Read the model definition and answer for the solid it produces. Units are mm, in the model's axes. A direction names the side the tool comes from. Coordinates: 2 decimals unless noted, no trailing zeros. Write each loop counter-clockwise with the first axis right and the second up, starting at its lowest first coordinate (ties: lowest second). Pieces come first, ordered by that corner, then holes.
1) Which of the six approach directions +Z, -Z, +X, -X, +Y, -Y give full straight-line access (tool end or side, diameter ignored) to faces 1 (the face through (0.301, 14.752, 0.285)), 2 (the face through (0.285, 4.248, 0.301)), 3 (the face through (1.875, 3.49, 3.127))?
2) The part is cut by section B-B (y = 9.5). Determine the outline of the cut face in (x, z), then the cut area to 3 significant figures.
3) The part is cut by section D-D (y = 16.25). Determine the outline of the cut face in (x, z), then the cut area to 3 significant figures.
4) The part is cut by section A-A (x = 30). Determine the outline of the cut face in (y, z).
5) The part is cut by section C-C (x = 12). Determine the outline of the cut face in (y, z), then the cut area to 3 significant figures.
6) Each of these flat-tipped pins is pushed along its axis until it touches: pin 1 Ø1.4 at (x, y) = (55, 3.5) entering from +Z; pin 2 Ø1.7 at (x, y) = (25, 14) entering from -Z. Where does it stop, or does it pass through?
7) Find the intervals of material crossed by line 1 (Y direction, x = 56, z = 2.4); line 2 (X direction, y = 13, z = 2.3); line 3 (Y direction, x = 54, z = 4.2), in increasing order.
8) Determine the mould class of faces 4 (the face through (45.875, 8.681, 3.127)), 5 (the face through (60, 9, 3)), 6 (the face through (30.392, 0.285, 0.301)) for opening direction X: +X half, -X half, draft (parallel to the pull), parting line (faces both ways), or undercut.
Autodesk Fusion 360 part; units mm, degrees
sketch "草图1" plane through (0, 0, 0) normal (0, 0, 1) x (1, 0, 0)
  line L0 (0, 0) -> (60, 0)
  line L1 (60, 0) -> (60, 19)
  line L2 (60, 19) -> (0, 19)
  line L3 (0, 19) -> (0, 0)
  line L4 (0, 9.5) -> (60, 9.5) construction
  line L5 (0, 12.44) -> (60, 12.44)
  line L6 (60, 12.44) -> (60, 6.56)
  line L7 (60, 6.56) -> (0, 6.56)
  line L8 (0, 6.56) -> (0, 12.44)
  line L9 (0, 12.44) -> (60, 6.56) construction
  line L10 (60, 12.44) -> (0, 6.56) construction
  point P0 (30, 9.5)
  point P1 (30, 9.5)
  dimension "d1" = 60
  dimension "d2" = 19
  dimension "d3" = 60
  dimension "d4" = 5.88
extrude "拉伸1" add sketch "草图1" along normal blind 5
extrude "拉伸2" add sketch "草图1" against normal blind 1 contours L1 L3 L5 L6 L7 L8
sketch "草图2" plane through (0, 0, 5) normal (0, 0, 1) x (-1, 0, 0)
  line L0 (0, 0) -> (-60, 0)
  line L1 (-60, 0) -> (-60, -19)
  line L2 (-60, -19) -> (0, -19)
  line L3 (0, -19) -> (0, 0)
  point P0 (-30, -9.5)
hole "孔1" at (30, 9.5, 5) direction (0, 0, -1) diameter 3.2 depth 8 tip angle 180 counterbore diameter 6.5 counterbore depth 3.4
sketch "草图4" plane through (0, 0, 5) normal (0, 0, 1) x (-1, 0, 0)
  circle A0 centre (-30, -9.5) radius 3.25
  line L0 (0, 0) -> (-60, 0)
  line L1 (-60, 0) -> (-60, -19)
  line L2 (-60, -19) -> (0, -19)
  line L3 (0, -19) -> (0, 0)
  line L4 (-40.689, -19) -> (-40.689, 3.3911)
  circle A1 centre (-56, -2.6) radius 2.3
  circle A2 centre (-56, -13) radius 2.3
  circle A3 centre (-48, -7.8) radius 2.3
  line L5 (-40.689, 3.3911) -> (-60, 3.3911)
  line L6 (-60, -19) -> (-40.689, -19)
  line L7 (-60, 3.3911) -> (-60, -19)
  line L8 (-19.311, -19) -> (0, -19)
  line L9 (-19.311, 3.3911) -> (-19.311, -19)
  line L10 (0, -19) -> (0, 3.3911)
  line L11 (0, 3.3911) -> (-19.311, 3.3911)
  circle A4 centre (-4, -2.6089) radius 2.3
  circle A5 centre (-12, -7.8089) radius 2.3
  circle A6 centre (-4, -13.0089) radius 2.3
  point P0 (-60, -19)
  point P1 (-60, -19)
  dimension "d14" = 4.6
  dimension "d15" = 4.6
  dimension "d16" = 4.6
  dimension "d17" = 4.6
  dimension "d18" = 4.6
  dimension "d19" = 4.6
extrude "拉伸3" cut sketch "草图4" against normal blind 3.8 contours A1 | A2 | A3 | A4 | A5 | A6
fillet "圆角1" radius 2 4 edges at (60, 0, 2.5) (60, 19, 2.5) (0, 19, 2.5) (0, 0, 2.5)
fillet "圆角2" radius 0.5 4 edges at (60, 9.5, -1) (30, 6.56, -1) (30, 12.44, -1) (0, 9.5, -1)
fillet "圆角3" radius 1 10 edges at (0, 4.28, 0) (0.5858, 0.5858, 0) (30, 0, 0) (59.4142, 0.5858, 0) (60, 4.28, 0) (60, 14.72, 0) (59.4142, 18.4142, 0) (30, 19, 0) (0.5858, 18.4142, 0) (0, 14.72, 0)
Reported:
1. face 1: -Z, -X, +Y
1. face 2: -Z, -X, -Y
1. face 3: +Z
2. outline: (0, -0.5) arc R0.5 ccw to (0.5, -1) - (28.4, -1) - (28.4, 1.6) - (26.75, 1.6) - (26.75, 5) - (13.56, 5) - (13.56, 1.2) - (10.44, 1.2) - (10.44, 5) - (0, 5) - close; (31.6, -1) - (59.5, -1) arc R0.5 ccw to (60, -0.5) - (60, 5) - (49.55, 5) - (49.55, 1.2) - (46.45, 1.2) - (46.45, 5) - (33.25, 5) - (33.25, 1.6) - (31.6, 1.6) - close
2. area: 306 mm2
3. outline: (0, 1) arc R1 ccw to (1, 0) - (59, 0) arc R1 ccw to (60, 1) - (60, 5) - (0, 5) - close
3. area: 300 mm2
4. outline: (0, 1) arc R1 ccw to (1, 0) - (6.56, 0) - (6.56, -0.5) arc R0.5 ccw to (7.06, -1) - (7.9, -1) - (7.9, 1.6) - (6.25, 1.6) - (6.25, 5) - (0, 5) - close; (11.1, -1) - (11.94, -1) arc R0.5 ccw to (12.44, -0.5) - (12.44, 0) - (18, 0) arc R1 ccw to (19, 1) - (19, 5) - (12.75, 5) - (12.75, 1.6) - (11.1, 1.6) - close
5. outline: (0, 1) arc R1 ccw to (1, 0) - (6.56, 0) - (6.56, -0.5) arc R0.5 ccw to (7.06, -1) - (11.94, -1) arc R0.5 ccw to (12.44, -0.5) - (12.44, 0) - (18, 0) arc R1 ccw to (19, 1) - (19, 5) - (10.11, 5) - (10.11, 1.2) - (5.51, 1.2) - (5.51, 5) - (0, 5) - close
5. area: 82.9 mm2
6. pin 1: stops at z = 1.2
6. pin 2: stops at z = 0
7. line 1: y = 0 to 0.3, 4.9 to 10.7, 15.3 to 19
7. line 2: x = 0 to 1.7, 6.3 to 53.7, 58.3 to 60
7. line 3: y = 0 to 1.46, 3.74 to 11.86, 14.14 to 19
8. face 4: undercut
8. face 5: +X half
8. face 6: draft
